Could you check a few things on this drawing? It's one solid part, dimensions in mm from its lowest x, y, z. A direction names the side the tool comes from. Coordinates: 2 decimals unless noted, no trailing zeros. Order: outer loops, then holes, each group sorted by start corner. A loop starts at its lowest first (then second) coordinate and runs counter-clockwise, first axis right, second up. Notation, with made-up numbers: (87.5, 43.25) -> (122.5, 43.25) arc R30 cw to (122.5, 78.25) -> close; hole circle Ø3 at (54.25, -39.5). An arc over 180 degrees is marked (long way). Use a Markdown table: item, result. Add a question column.
1. For pin 1 Ø3 at (x, z) = (45, 46) entering from +Y; pin 2 Ø6.5 at (x, z) = (52.31, 11.25) entering from -Y; pin 3 Ø1 at (x, y) = (48, 15.5) entering from -Z; pin 4 Ø2 at (y, z) = (28, 12.5) entering from +X, each with a flat end and sliding along its axis, tell me the tip position at first contact or that it passes through.
2. For the marked faces 1 and 2, which set-ups out of +Z, -Z, +X, -X, +Y, -Y let a thin tool reach every point of the face, with its end or its side?
3. If I drill on line 1 along X through (y, z) = (4, 46); line 2 along X through (y, z) = (3, 12); line 3 along Y through (x, z) = (34.5, 53), over which ranges is the centre line in solid material (lowest first)? Write a range as from..to.
4. Suppose I cut it at B-B, the plane y = 41. List the corners of the cut face in (x, z) for me.
5. Suppose I cut it at A-A, the plane z = 55. List the corners of the cut face in (x, y) for me, then the cut area to 3 significant figures.
6. Suppose I cut it at C-C, the plane x = 16. State how many separate pieces and enclosed holes the cut face has, then the cut area to 3 significant figures.
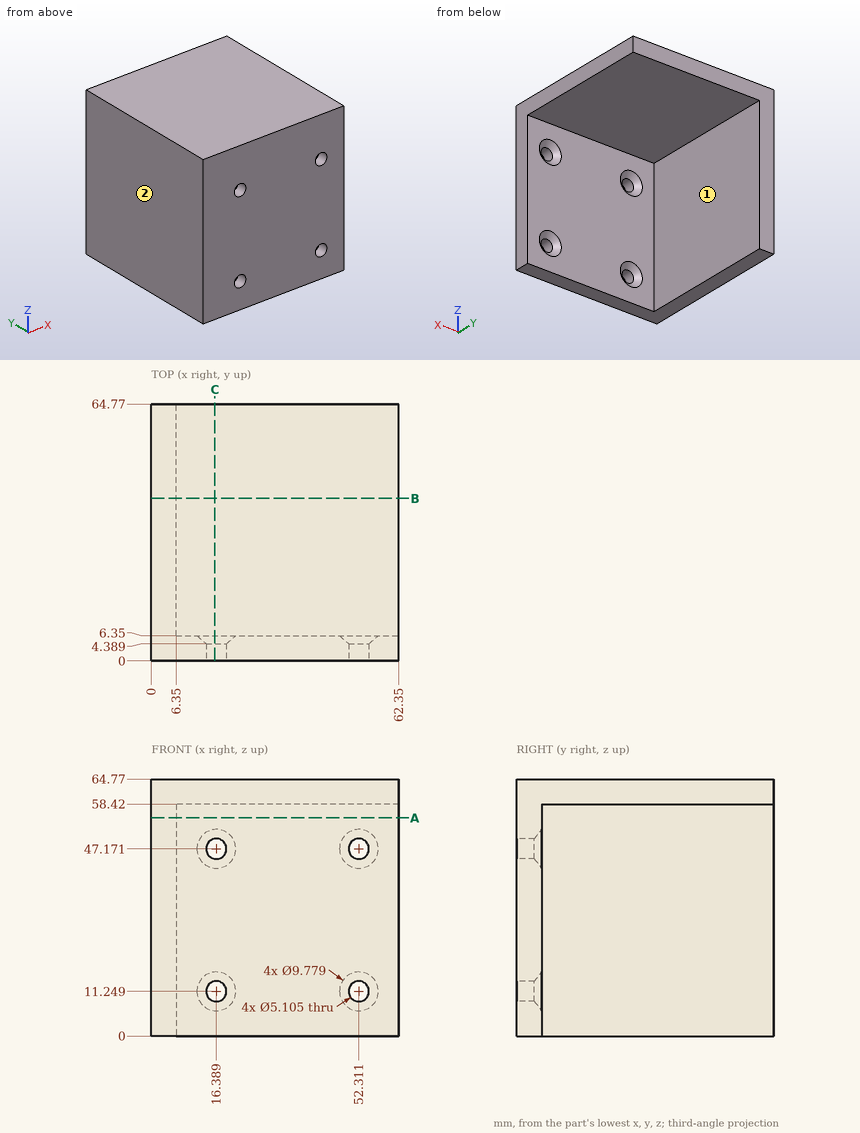
Worked out:
| question | item | result |
|---|---|---|
| 1 | pin 1 | stops at y = 6.35 |
| 1 | pin 2 | stops at y = 0 |
| 1 | pin 3 | stops at z = 58.42 |
| 1 | pin 4 | stops at x = 6.35 |
| 2 | face 1 | -Z, +X, +Y |
| 2 | face 2 | +Z, -Z, -X, +Y, -Y |
| 3 | line 1 | x = 0..14.12, 18.66..50.04, 54.58..62.35 |
| 3 | line 2 | x = 0..13.95, 18.83..49.87, 54.75..62.35 |
| 3 | line 3 | y = 0..6.35 |
| 4 | outline | (0, 0) -> (6.35, 0) -> (6.35, 58.42) -> (62.35, 58.42) -> (62.35, 64.77) -> (0, 64.77) -> close |
| 5 | outline | (0, 0) -> (62.35, 0) -> (62.35, 6.35) -> (6.35, 6.35) -> (6.35, 64.77) -> (0, 64.77) -> close |
| 5 | area | 767 mm² |
| 6 | separate pieces | 3 |
| 6 | enclosed holes | 0 |
| 6 | area | 709 mm² |
